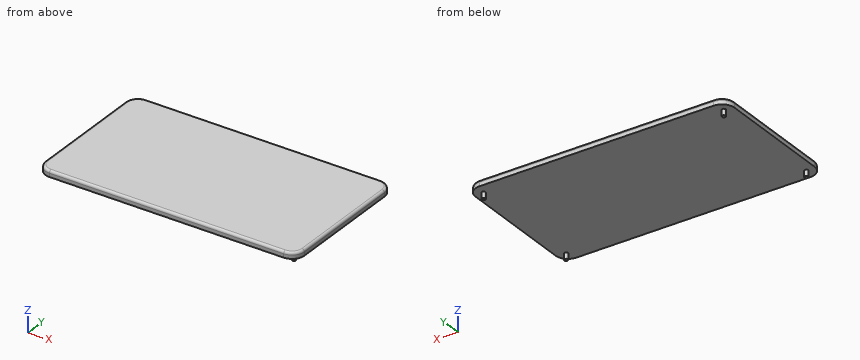
Autodesk Fusion 360 part; units mm, degrees
sketch "Sketch1" plane through (0, 0, 0) normal (0, 0, 1) x (1, 0, 0)
  line L0 (105, 57.5) -> (-105, 57.5)
  line L1 (-105, 57.5) -> (-105, -57.5)
  line L2 (-105, -57.5) -> (105, -57.5)
  line L3 (105, -57.5) -> (105, 57.5)
  line L4 (105, 57.5) -> (-105, -57.5) construction
  line L5 (-105, 57.5) -> (105, -57.5) construction
  circle A0 centre (97.5, -49) radius 1.5
  line L6 (0, 57.5) -> (0, -57.5) construction
  line L7 (-105, 0) -> (105, 0) construction
  circle A1 centre (97.5, 49) radius 1.5
  circle A2 centre (-97.5, -49) radius 1.5
  circle A3 centre (-97.5, 49) radius 1.5
  dimension "d1" = 210
  dimension "d2" = 115
  dimension "d3" = 3
  dimension "d4" = 97.5
  dimension "d5" = 49
extrude "Extrude1" add sketch "Sketch1" along normal blind 5 contours L0 L1 L2 L3 | A0 | A1 | A2 | A3
extrude "Extrude2" add sketch "Sketch1" against normal blind 5 contours A0 | A1 | A2 | A3
fillet "Fillet1" radius 10 4 edges at (-105, -57.5, 2.5) (-105, 57.5, 2.5) (105, -57.5, 2.5) (105, 57.5, 2.5)
fillet "Fillet2" radius 2 8 edges at (102.0711, -54.5711, 5) (105, 0, 5) (102.0711, 54.5711, 5) (0, 57.5, 5) (-102.0711, 54.5711, 5) (-105, 0, 5) (-102.0711, -54.5711, 5) (0, -57.5, 5)
equation "d4 = ( 195 / 2 ) * 1 mm"
equation "d5 = ( 98 / 2 ) * 1 mm"
Design review of the part built by this model. Coordinates are the model's own, in mm. Round coordinates to 2 decimals unless told otherwise and drop trailing zeros. Loops run counter-clockwise (first coordinate to the right, second up) from the corner with the lowest first, then second, coordinate; pieces in that order, holes last. Notation, with made-up numbers: M 57.5,42.25 L 112.5,42.25 A32 cw 112.5,72.25 Z; hole C 32.5,61 d10. An arc over 180 degrees is marked long. Answer as a JSON object with one key per item and string values.
Item 1: We need section B-B on y = -41. Give the boundary of the cut face in (x, z), and give its area (3 significant figures).
Answer sheet:
{"outline": "M -105,0 L 105,0 L 105,3 A2 ccw 103,5 L -103,5 A2 ccw -105,3 Z", "area": "1,050 mm^2"}
Item 2: We need section A-A on x = 47.5. Give the boundary of the cut face in (y, z), and give its area (3 significant figures).
Answer sheet:
{"outline": "M -57.5,0 L 57.5,0 L 57.5,3 A2 ccw 55.5,5 L -55.5,5 A2 ccw -57.5,3 Z", "area": "573 mm^2"}
Item 3: Clearance check with flat-ended pins moving along their axes: P1, Ø1.5, axis at x = 17, z = -2, coming from the -Y side; P2, Ø8, axis at x = 46.5, y = 41, coming from the -Z side. State where each tip first meets the part, or that it passes through.
Answer sheet:
{"P1": "passes through", "P2": "stops at z = 0"}
Item 4: Wall thickness on L1, parallel to Z at x = 86, y = 25; L2, parallel to Y at x = 32, z = 4.75; L3, parallel to X at y = 17.5, z = 4.5: over which ranges is each line inside the solid? List them lowest first. Write a range as from..to.
Answer sheet:
{"L1": "z = 0..5", "L2": "y = -56.47..56.47", "L3": "x = -104.32..104.32"}
Item 5: We need section C-C on z = -2.25. Give the boundary of the cut face in (x, y).
Answer sheet:
{"outline": "C -97.5,-49 d3; C -97.5,49 d3; C 97.5,-49 d3; C 97.5,49 d3"}
